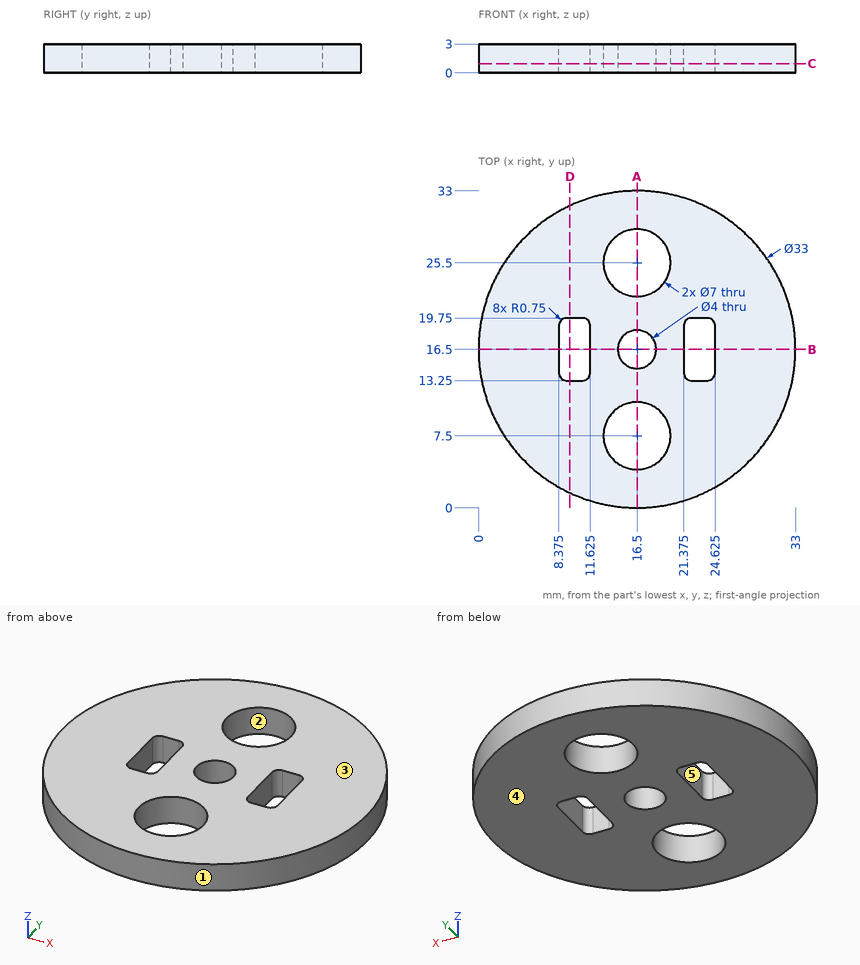
Design review of the part shown in the three views and the two pictorial views. Dimensions are in mm from the part's minimum x, y and z. A direction names the side the tool comes from. Round coordinates to 2 decimals unless told otherwise and drop trailing zeros. Loops run counter-clockwise (first coordinate to the right, second up) from the corner with the lowest first, then second, coordinate; pieces in that order, holes last.
Q1. Add section D-D on x = 9.5. Write out the cut boundary in (y, z), plus the area to 3 significant figures.
Result sheet:
outline: (1.56, 0) - (13.25, 0) - (13.25, 3) - (1.56, 3) - close; (19.75, 0) - (31.44, 0) - (31.44, 3) - (19.75, 3) - close
area: 70.1 mm2
Q2. Insertion check: pin 1 Ø1.5 at (y, z) = (26.5, 0.5) entering from +X; pin 2 Ø11 at (x, y) = (16.5, 7.5) entering from +Z; pin 3 Ø1.5 at (x, z) = (4, 2.5) entering from +Y; pin 4 Ø0.5 at (x, z) = (9.5, 1.5) entering from +Y. Each pin has a flat end and moves straight along its axis. Give the tip position at first contact, or say it passes through.
Result sheet:
pin 1: stops at x = 30.16
pin 2: stops at z = 3
pin 3: stops at y = 28.08
pin 4: stops at y = 31.56
Q3. Add section B-B on y = 16.5. Write out the cut boundary in (x, z) (3 decimals), plus the area to 3 significant figures.
Result sheet:
outline: (0, 0) - (8.375, 0) - (8.375, 3) - (0, 3) - close; (11.625, 0) - (14.5, 0) - (14.5, 3) - (11.625, 3) - close; (18.5, 0) - (21.375, 0) - (21.375, 3) - (18.5, 3) - close; (24.625, 0) - (33, 0) - (33, 3) - (24.625, 3) - close
area: 67.5 mm2
Q4. Mouldability with a two-part tool opening along X and no side actions: class the marked faces 1, 2 and 3 as +X half, -X half, draft (parallel to the pull), parting line (faces both ways), or undercut.
Result sheet:
face 1: parting line
face 2: undercut
face 3: draft
Q5. Machinability: for the marked faces 4 and 5, which of the approach directions +Z, -Z, +X, -X, +Y, -Y give a long, thin tool a straight path to every point of the face, cutting with its end or side? Answer none if there is none.
Result sheet:
face 4: -Z, +X, -X, +Y, -Y
face 5: +Z, -Z
Q6. Add section C-C on z = 0.95. Write out the cut boundary in (x, y) (3 decimals), plus the area to 3 significant figures.
Result sheet:
outline: circle Ø33 at (16.5, 16.5); hole (8.375, 14) arc R0.75 ccw to (9.125, 13.25) - (10.875, 13.25) arc R0.75 ccw to (11.625, 14) - (11.625, 19) arc R0.75 ccw to (10.875, 19.75) - (9.125, 19.75) arc R0.75 ccw to (8.375, 19) - close; hole circle Ø7 at (16.5, 7.5); hole circle Ø7 at (16.5, 25.5); hole circle Ø4 at (16.5, 16.5); hole (21.375, 14) arc R0.75 ccw to (22.125, 13.25) - (23.875, 13.25) arc R0.75 ccw to (24.625, 14) - (24.625, 19) arc R0.75 ccw to (23.875, 19.75) - (22.125, 19.75) arc R0.75 ccw to (21.375, 19) - close
area: 724 mm2
Q7. To check wall thickness, follow line 1 along Y through (x, z) = (16.5, 1.7); line 2 along Y through (x, z) = (17.5, 1.1); line 3 along X through (y, z) = (22.5, 2.65). State the ranges of each line that lie inside material, in increasing order.
Result sheet:
line 1: y = 0 to 4, 11 to 14.5, 18.5 to 22, 29 to 33
line 2: y = 0.03 to 4.15, 10.85 to 14.77, 18.23 to 22.15, 28.85 to 32.97
line 3: x = 1.13 to 14.7, 18.3 to 31.87
Q8. Add section A-A on x = 16.5. Write out the cut boundary in (y, z), plus the area to 3 significant figures.
Result sheet:
outline: (0, 0) - (4, 0) - (4, 3) - (0, 3) - close; (11, 0) - (14.5, 0) - (14.5, 3) - (11, 3) - close; (18.5, 0) - (22, 0) - (22, 3) - (18.5, 3) - close; (29, 0) - (33, 0) - (33, 3) - (29, 3) - close
area: 45.0 mm2
